The figure shows three views and two pictorial views of one solid part (mm, origin at its lowest corner). Answer the questions. Round coordinates to 2 decimals unless told otherwise and drop trailing zeros. Order: outer loops, then holes, each group sorted by start corner. A loop starts at its lowest first (then second) coordinate and runs counter-clockwise, first axis right, second up.
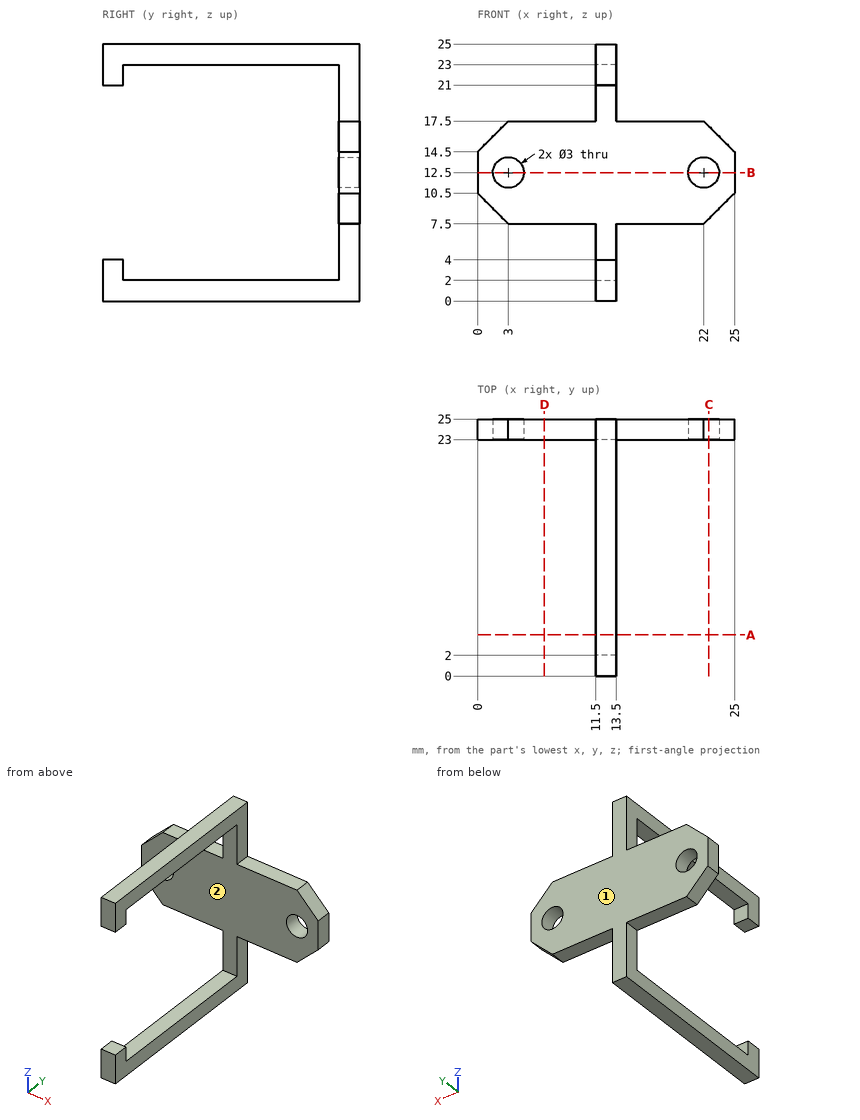
Item 1: Find section D-D (x = 6.5). Write down the section's boundary in (y, z), plus the area to 3 significant figures.
Item 2: Find section C-C (x = 22.5). Write down the section's boundary in (y, z).
Item 3: Find the intervals of material crossed by line 1 along X through (y, z) = (23.7, 12.5); line 2 along Z through (x, y) = (12.25, 21); line 3 along Y through (x, z) = (15.75, 15.75), in increasing order.
Item 4: Find section A-A (y = 4). Write down the section's boundary in (x, z), plus the area to 3 significant figures.
Item 5: Find section B-B (z = 12.5). Write down the section's boundary in (x, y).
Item 6: Given pin 1 (12 mm diameter, centred on y = 8.5, z = 6.5, fed in from -X); pin 2 (3.5 mm diameter, centred on x = 22, z = 12.5, fed in from -Y); pin 3 (0.6 mm diameter, centred on x = 9.5, y = 24, fed in from +Z); pin 4 (4 mm diameter, centred on y = 16.5, z = 4.5, fed in from -X), each flat-ended and moving along its own axis, determine where each tip first touches the part or whether it passes through.
Item 7: For a pull along Z with two mould halves and no side action, classify the marked faces 1 and 2 as released by +Z, released by -Z, zero draft, split by the parting line, or undercut.
Model answer:
1. outline: (23, 7.5) - (25, 7.5) - (25, 17.5) - (23, 17.5) - close
1. area: 20.0 mm2
2. outline: (23, 8) - (25, 8) - (25, 11.09) - (23, 11.09) - close; (23, 13.91) - (25, 13.91) - (25, 17) - (23, 17) - close
3. line 1: x = 0 to 1.5, 4.5 to 20.5, 23.5 to 25
3. line 2: z = 0 to 2, 23 to 25
3. line 3: y = 23 to 25
4. outline: (11.5, 0) - (13.5, 0) - (13.5, 2) - (11.5, 2) - close; (11.5, 23) - (13.5, 23) - (13.5, 25) - (11.5, 25) - close
4. area: 8.00 mm2
5. outline: (0, 23) - (1.5, 23) - (1.5, 25) - (0, 25) - close; (4.5, 23) - (20.5, 23) - (20.5, 25) - (4.5, 25) - close; (23.5, 23) - (25, 23) - (25, 25) - (23.5, 25) - close
6. pin 1: stops at x = 11.5
6. pin 2: stops at y = 23
6. pin 3: stops at z = 17.5
6. pin 4: passes through
7. face 1: zero draft
7. face 2: undercut
